Input: part model. Units: mm. Frame: model coordinates. A direction names the side the tool comes from. Coordinates: 2 decimals unless noted, no trailing zeros. Loops run counter-clockwise (first coordinate to the right, second up) from the corner with the lowest first, then second, coordinate; pieces in that order, holes last.
Item 1: Section D-D on y = -1.25. Return loops of the section in (x, z).
Item 2: Section A-A on x = -1. Return loops of the section in (y, z).
Item 3: Ray query, line 1 along Y through (x, z) = (35.91, 2.65); line 2 along X through (y, z) = (-2.25, 1.8); line 3 along Y through (x, z) = (1, 0.85). Return the intervals inside material, ascending.
Item 4: Contact query for flat-ended pins moving along their axis: P1, Ø0.7, axis at y = -1, z = 1.5, coming from the +X side; P2, Ø0.8, axis at y = 3, z = 1.5, coming from the -X side; P3, Ø1.5, axis at y = 2.5, z = 3.5, coming from the +X side. Output: stop coordinate, or through.
Item 5: Section C-C on x = 23.5. Return loops of the section in (y, z), and give its area (3 significant figures).
Item 6: Reachability of faces 4 (the cylindrical face through (11.61, 5.66, 2.71)), 5 (the flat face through (-3, 0, 2.3)), 6 (the flat face through (18.468, -3, 2)), 7 (the flat face through (19.624, 3, 2)) from +Z, -Z, +X, -X, +Y, -Y: full face, straight path, thin tool, end or side. Return the list, or none.
Item 7: Pull-direction query (X, two-part tool) for faces 1 (the flat face through (7.41, -6.5, 2.7)), 2 (the flat face through (35.7, -4, 2.7)), 3 (the flat face through (33.366, 0, 2)); classes: released by +X, released by -X, zero draft, split by the parting line, or undercut.
```python
from build123d import *

# Parameters (mm, degrees)
ESQUISSE1_W             = 14.82
ESQUISSE1_H             = 12
BOSS_EXTRU_1_DEPTH      = 4.5
ESQUISSE2_W             = 2
ESQUISSE2_H             = 11.4
ENL_V_MAT_EXTRU_1_DEPTH = 9
CONG_1_R                = 0.2
ESQUISSE3_W             = 30
ESQUISSE3_H             = 14
BOSS_EXTRU_2_DEPTH      = 0.9
ENL_V_MAT_EXTRU_2_REACH = 6.5
ESQUISSE4_W             = 2
ESQUISSE4_H             = 2.5
ESQUISSE5_R             = 0.7
ESQUISSE5_W             = 3.3
ESQUISSE5_H             = 8
ENL_V_MAT_EXTRU_3_DEPTH = 4.15
ESQUISSE6_W             = 20
ESQUISSE6_H             = 12.2
BOSS_EXTRU_3_DEPTH      = 1.3
ESQUISSE7_W             = 8.197434371
ESQUISSE7_H             = 6.831195309
ESQUISSE7_W_2           = 1.366239062
ESQUISSE7_H_2           = 2.101906249
ESQUISSE7_W_3           = 1.261143749
ESQUISSE7_W_4           = 2.522287499
ESQUISSE7_H_3           = 1.050953124
ESQUISSE7_W_5           = 0.570374351
ESQUISSE7_H_4           = 1.05519255
BOSS_EXTRU_4_DEPTH      = 1.4
ESQUISSE8_W             = 4
ESQUISSE8_H             = 10
BOSS_EXTRU_5_DEPTH      = 2.25
ESQUISSE9_W             = 1.2
ESQUISSE9_H             = 1.35
ENL_V_MAT_EXTRU_4_DEPTH = 4.15


with BuildPart() as part:
    # Esquisse1 → Boss.-Extru.1 (new body)
    with BuildSketch(Plane.XY):
        Rectangle(ESQUISSE1_W, ESQUISSE1_H)
    extrude(amount=BOSS_EXTRU_1_DEPTH)

    # Esquisse2 → Enlèv. mat.-Extru.1 (cut)
    with BuildSketch(Plane.ZY.offset(7.41)):
        with Locations((1.3, 0)):
            Rectangle(ESQUISSE2_W, ESQUISSE2_H)
    extrude(amount=-ENL_V_MAT_EXTRU_1_DEPTH, mode=Mode.SUBTRACT)

    # Congé1
    cong_1_edges = [part.edges().sort_by_distance(p)[0] for p in [
        (0, -6, 4.5),
        (0, -6, 0),
        (0, 6, 0),
        (0, 6, 4.5),
    ]]
    fillet(cong_1_edges, radius=CONG_1_R)

    # Esquisse3 → Boss.-Extru.2 (add)
    with BuildSketch(Plane.XY.offset(2.25)):
        with Locations((22.41, 0)):
            Rectangle(ESQUISSE3_W, ESQUISSE3_H)
    extrude(amount=BOSS_EXTRU_2_DEPTH)

    # Esquisse4 → Enlèv. mat.-Extru.2 (cut, up to next)
    with BuildSketch(Plane(origin=(0, 0, 0), x_dir=(-1, 0, 0), z_dir=(0, 0, -1)), mode=Mode.PRIVATE) as enl_v_mat_extru_2_sk1:
        with Locations((1.41, 2.95)):
            Rectangle(ESQUISSE4_W, ESQUISSE4_H)
    enl_v_mat_extru_2_tool1 = extrude(enl_v_mat_extru_2_sk1.sketch, amount=-ENL_V_MAT_EXTRU_2_REACH, mode=Mode.PRIVATE) & part.part
    add(enl_v_mat_extru_2_tool1.solids().sort_by_distance((-1.41, 2.95, 0))[0], mode=Mode.SUBTRACT)
    # Esquisse4 → Enlèv. mat.-Extru.2 (cut, up to next)
    with BuildSketch(Plane(origin=(0, 0, 0), x_dir=(-1, 0, 0), z_dir=(0, 0, -1)), mode=Mode.PRIVATE) as enl_v_mat_extru_2_sk2:
        with Locations((1.41, -2.95)):
            Rectangle(ESQUISSE4_W, ESQUISSE4_H)
    enl_v_mat_extru_2_tool2 = extrude(enl_v_mat_extru_2_sk2.sketch, amount=-ENL_V_MAT_EXTRU_2_REACH, mode=Mode.PRIVATE) & part.part
    add(enl_v_mat_extru_2_tool2.solids().sort_by_distance((-1.41, -2.95, 0))[0], mode=Mode.SUBTRACT)

    # Esquisse5 → Enlèv. mat.-Extru.3 (cut, through all)
    with BuildSketch(Plane.XY.offset(3.15)):
        with Locations((35.91, 5.4)):
            Circle(ESQUISSE5_R)
        with Locations((35.91, -5.4)):
            Circle(ESQUISSE5_R)
        with Locations((35.76, 0)):
            Rectangle(ESQUISSE5_W, ESQUISSE5_H)
        with BuildLine():
            Line((9.81, 6.25), (11.01, 6.25))
            ThreePointArc((11.01, 6.25), (11.61, 5.65), (11.01, 5.05))
            Line((11.01, 5.05), (9.81, 5.05))
            ThreePointArc((9.81, 5.05), (9.21, 5.65), (9.81, 6.25))
        make_face()
        with BuildLine():
            Line((9.81, -6.25), (11.01, -6.25))
            ThreePointArc((11.01, -6.25), (11.61, -5.65), (11.01, -5.05))
            Line((11.01, -5.05), (9.81, -5.05))
            ThreePointArc((9.81, -5.05), (9.21, -5.65), (9.81, -6.25))
        make_face()
    extrude(amount=-ENL_V_MAT_EXTRU_3_DEPTH, mode=Mode.SUBTRACT)

    # Esquisse6 → Boss.-Extru.3 (add)
    with BuildSketch(Plane.XY.offset(3.15)):
        with Locations((23.41, 0)):
            Rectangle(ESQUISSE6_W, ESQUISSE6_H)
    extrude(amount=BOSS_EXTRU_3_DEPTH)

    # Esquisse7 → Boss.-Extru.4 (add)
    with BuildSketch(Plane(origin=(0, 0, 2.25), x_dir=(-1, 0, 0), z_dir=(0, 0, -1))):
        with Locations((-26.770674994, -0.052547657)):
            Rectangle(ESQUISSE7_W, ESQUISSE7_H)
        with Locations((-17.78502578, -3.257954686)):
            Rectangle(ESQUISSE7_W_2, ESQUISSE7_H_2)
        with Locations((-14.684714062, -3.257954686)):
            Rectangle(ESQUISSE7_W_3, ESQUISSE7_H_2)
        with Locations((-18.363049999, 2.837573436)):
            Rectangle(ESQUISSE7_W_4, ESQUISSE7_H_3)
        with Locations((-33.651427146, -0.16121887)):
            Rectangle(ESQUISSE7_W_5, ESQUISSE7_H_4)
    extrude(amount=BOSS_EXTRU_4_DEPTH)

    # Esquisse8 → Boss.-Extru.5 (add)
    with BuildSketch(Plane(origin=(0, 0, 2.25), x_dir=(-1, 0, 0), z_dir=(0, 0, -1))):
        with Locations((-9.41, 0)):
            Rectangle(ESQUISSE8_W, ESQUISSE8_H)
    extrude(amount=BOSS_EXTRU_5_DEPTH)

    # Esquisse9 → Enlèv. mat.-Extru.4 (cut, through all)
    with BuildSketch(Plane.XY.offset(3.15)):
        with Locations((9.81, 6.325)):
            Rectangle(ESQUISSE9_W, ESQUISSE9_H)
        with Locations((9.81, -6.325)):
            Rectangle(ESQUISSE9_W, ESQUISSE9_H)
    extrude(amount=-ENL_V_MAT_EXTRU_4_DEPTH, mode=Mode.SUBTRACT)


solid = part.part
```
Results found:
1. outline: (-7.41, 0) - (11.41, 0) - (11.41, 2.25) - (22.67, 2.25) - (22.67, 0.85) - (30.87, 0.85) - (30.87, 2.25) - (34.11, 2.25) - (34.11, 3.15) - (33.41, 3.15) - (33.41, 4.45) - (13.41, 4.45) - (13.41, 3.15) - (7.41, 3.15) - (7.41, 4.5) - (-7.41, 4.5) - (-7.41, 2.3) - (1.59, 2.3) - (1.59, 0.3) - (-7.41, 0.3) - close
2. outline: (-6, 0.2) arc R0.2 ccw to (-5.8, 0) - (-4.2, 0) - (-4.2, 0.3) - (-5.7, 0.3) - (-5.7, 2.3) - (5.7, 2.3) - (5.7, 0.3) - (4.2, 0.3) - (4.2, 0) - (5.8, 0) arc R0.2 ccw to (6, 0.2) - (6, 4.3) arc R0.2 ccw to (5.8, 4.5) - (-5.8, 4.5) arc R0.2 ccw to (-6, 4.3) - close; (-1.7, 0) - (1.7, 0) - (1.7, 0.3) - (-1.7, 0.3) - close
3. line 1: y = -7 to -6.1, -4.7 to -4, 4 to 4.7, 6.1 to 7
3. line 2: x = 1.59 to 11.41, 14.05 to 15.32, 17.1 to 18.47, 22.67 to 30.87
3. line 3: y = -6 to -5.7, 5.7 to 6
4. P1: stops at x = 33.94
4. P2: stops at x = 1.59
4. P3: stops at x = 34.11
5. outline: (-7, 2.25) - (-3.47, 2.25) - (-3.47, 0.85) - (3.36, 0.85) - (3.36, 2.25) - (7, 2.25) - (7, 3.15) - (6.1, 3.15) - (6.1, 4.45) - (-6.1, 4.45) - (-6.1, 3.15) - (-7, 3.15) - close
5. area: 38.0 mm2
6. face 4: +Z, -Z
6. face 5: -X
6. face 6: -Z, -Y
6. face 7: -Z, +Y, -Y
7. face 1: released by -X
7. face 2: zero draft
7. face 3: undercut
